Geometry: final body of the model. Coordinates: model frame, mm. Give positions to 0.01 mm unless a question says otherwise; leave off trailing zeros. Loops run counter-clockwise (first coordinate to the right, second up) from the corner with the lowest first, then second, coordinate; pieces in that order, holes last.
Autodesk Inventor part; units mm, degrees
ref_plane "YZ Plane" through (0, 0, 0) normal (1, 0, 0) x (0, 1, 0)
ref_plane "XZ Plane" through (0, 0, 0) normal (0, 1, 0) x (-1, 0, 0)
ref_plane "XY Plane" through (0, 0, 0) normal (0, 0, 1) x (1, 0, 0)
sketch "Esquisse1" plane through (0, 0, 0) normal (0, 1, 0) x (-1, 0, 0)
  line L0 (0, 0) -> (25, 0)
  line L1 (25, 0) -> (0, 0)
  line L2 (0, 0) -> (0, 9)
  line L3 (0, 9) -> (25, 0)
  arc A0 (25, 0) -> (15, 0) centre (20, 0) ccw
  dimension "d0" = 9
  dimension "d1" = 25
  dimension "d2" = 5
revolve "Révolution1" add sketch "Esquisse1" angle 360 about axis through (-25, 0, 0) along (1, 0, 0)
sketch "Esquisse2" plane through (0, 0, 0) normal (1, 0, 0) x (0, 0, -1)
  line L0 (-0.3714, 0.9357) -> (0.3286, 0.9357)
  line L1 (0.3286, 0.9357) -> (0.3286, -0.9643)
  line L2 (0.3286, -0.9643) -> (-0.3714, -0.9643)
  line L3 (-0.3714, -0.9643) -> (-0.3714, 0.9357)
  line L4 (0.9286, 0.3357) -> (-0.9714, 0.3357)
  line L5 (-0.9714, 0.3357) -> (-0.9714, -0.3643)
  line L6 (-0.9714, -0.3643) -> (0.9286, -0.3643)
  line L7 (0.9286, -0.3643) -> (0.9286, 0.3357)
  point P0 (0, 0)
  dimension "d4" = 0.7
  dimension "d5" = 0.7
  dimension "d6" = 1.9
  dimension "d7" = 1.9
  dimension "d8" = 0.6
  dimension "d9" = 0.6
extrude "Extrusion1" cut sketch "Esquisse2" against normal blind 10
properties part number "pion" material "Verre"
Item 1: Section query C-C on y = 0. Return loops of the section in (x, z).
Values follow:
outline: (-16.15, -3.19) - (0, -9) - (0, -0.93) - (-10, -0.93) - (-10, 0.97) - (0, 0.97) - (0, 9) - (-16.15, 3.19) arc R5 ccw (long way) to start
Item 2: Section query D-D on x = -7. Return loops of the section in (y, z).
Values follow:
outline: circle Ø12.96 at (0, 0); hole (-0.96, -0.33) - (-0.36, -0.33) - (-0.36, -0.93) - (0.34, -0.93) - (0.34, -0.33) - (0.94, -0.33) - (0.94, 0.37) - (0.34, 0.37) - (0.34, 0.97) - (-0.36, 0.97) - (-0.36, 0.37) - (-0.96, 0.37) - close
Item 3: Section query B-B on z = 0. Return loops of the section in (x, y).
Values follow:
outline: (-16.15, -3.19) - (0, -9) - (0, -0.96) - (-10, -0.96) - (-10, 0.94) - (0, 0.94) - (0, 9) - (-16.15, 3.19) arc R5 ccw (long way) to start
Item 4: Pin query (flat end, axial travel): pin 1 (0.5 mm diameter, centred on x = -6.5, y = -0.5, fed in from +Z); pin 2 (0.7 mm diameter, centred on x = -5.5, z = 0.5, fed in from +Y); pin 3 (1.5 mm diameter, centred on x = -13, y = -2, fed in from +Z). Return the tip coordinate at first contact, or that it passes through.
Values follow:
pin 1: stops at z = 6.73
pin 2: stops at y = 7.13
pin 3: stops at z = 4.27
Item 5: Ray query, probe 1 along Z at (x, y) = (-7, 0.75); probe 2 along Z at (x, y) = (-6, -2); probe 3 along X at (y, z) = (-3.75, -6). Return the intervals inside material, ascending.
Values follow:
probe 1: z = -6.44 to -0.33, 0.37 to 6.44
probe 2: z = -6.54 to 6.54
probe 3: x = -5.35 to 0
Item 6: Draft query along Z for faces 1 (the face through (-10, 0, 0)), 2 (the face through (-9.755, -0.241, -5.483)), 3 (the face through (0, 2, 0)). Return one class per face: +Z half, -Z half, draft (parallel to the pull), parting line (faces both ways), or undercut.
Values follow:
face 1: undercut
face 2: parting line
face 3: draft
Item 7: Section query A-A on x = -2. Return loops of the section in (y, z), plus the area to 3 significant figures.
Values follow:
outline: circle Ø16.56 at (0, 0); hole (-0.96, -0.33) - (-0.36, -0.33) - (-0.36, -0.93) - (0.34, -0.93) - (0.34, -0.33) - (0.94, -0.33) - (0.94, 0.37) - (0.34, 0.37) - (0.34, 0.97) - (-0.36, 0.97) - (-0.36, 0.37) - (-0.96, 0.37) - close
area: 213 mm2
